Design review of the part shown in the three views and the two pictorial views. Dimensions are in mm from the part's minimum x, y and z. A direction names the side the tool comes from. Round coordinates to 2 decimals unless told otherwise and drop trailing zeros. Write each loop counter-clockwise with the first axis right and the second up, starting at its lowest first coordinate (ties: lowest second). Pieces come first, ordered by that corner, then holes. Notation, with made-up numbers: (25, 8) -> (83, 8) arc R24 cw to (83, 20) -> close; hole circle Ø4 at (8.5, 81.25). An arc over 180 degrees is marked (long way). Return JSON: item names as keys, results as strings. Group by question number.
1. Take a section at A-A, the plane z = 532.5. Write out the cut boundary in (x, y), then the cut area to 3 significant figures.
2. Take a section at D-D, the plane z = 832.5. Write out the cut boundary in (x, y), then the cut area to 3 significant figures.
3. Take a section at B-B, the plane y = 568.5. Write out the cut boundary in (x, z), then the cut area to 3 significant figures.
4. Clearance check with flat-ended pins moving along their axes: P1, Ø23, axis at x = 125.5, z = 437.5, coming from the +Y side; P2, Ø23, axis at y = 121.5, z = 427, coming from the -X side. State where each tip first meets the part, or that it passes through.
5. Mouldability with a two-part tool opening along Y and no side actions: class the marked faces 1, 2 and 3 as pulls with the +Y half, pulls with the -Y half, needs draft (parallel to the pull), parting line crosses it, or undercut.
6. Tool access review of the marked faces 4 and 5: name each direction out of +Z, -Z, +X, -X, +Y, -Y from which nothing blocks a thin tool from reaching the whole face with its end or side.
7. For line 1 along X through (y, z) = (1194, 764); line 2 along Y through (x, z) = (2033, 168); line 3 along X through (y, z) = (141, 113), list the stretches that pass through material, from the lowest coordinate up. Write a range as from..to.
8. Take a section at C-C, the plane x = 857. Write out the cut boundary in (y, z), then the cut area to 3 significant figures.
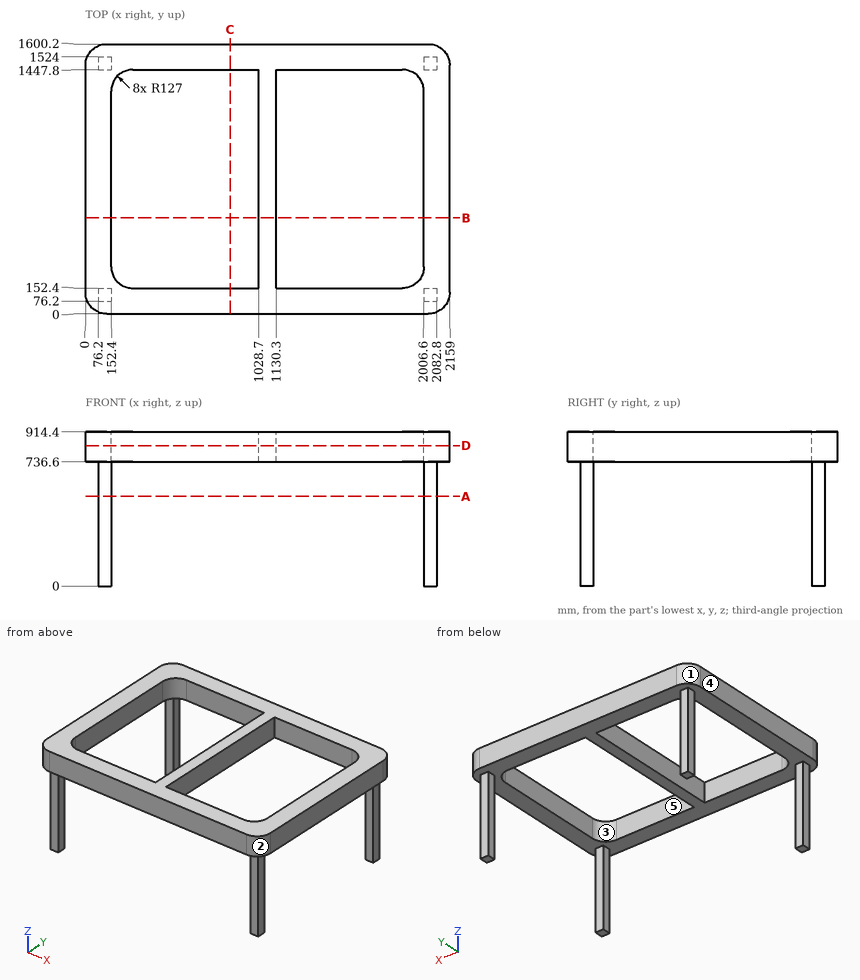
Output:
{
 "1": {"outline": "(76.2, 76.2) -> (152.4, 76.2) -> (152.4, 152.4) -> (76.2, 152.4) -> close; (76.2, 1447.8) -> (152.4, 1447.8) -> (152.4, 1524) -> (76.2, 1524) -> close; (2006.6, 76.2) -> (2082.8, 76.2) -> (2082.8, 152.4) -> (2006.6, 152.4) -> close; (2006.6, 1447.8) -> (2082.8, 1447.8) -> (2082.8, 1524) -> (2006.6, 1524) -> close", "area": "23,200 mm^2"},
 "2": {"outline": "(0, 127) arc R127 ccw to (127, 0) -> (2032, 0) arc R127 ccw to (2159, 127) -> (2159, 1473.2) arc R127 ccw to (2032, 1600.2) -> (127, 1600.2) arc R127 ccw to (0, 1473.2) -> close; hole (152.4, 279.4) arc R127 ccw to (279.4, 152.4) -> (1028.7, 152.4) -> (1028.7, 1447.8) -> (279.4, 1447.8) arc R127 ccw to (152.4, 1320.8) -> close; hole (1130.3, 152.4) -> (1879.6, 152.4) arc R127 ccw to (2006.6, 279.4) -> (2006.6, 1320.8) arc R127 ccw to (1879.6, 1447.8) -> (1130.3, 1447.8) -> close", "area": "1,180,000 mm^2"},
 "3": {"outline": "(0, 736.6) -> (152.4, 736.6) -> (152.4, 914.4) -> (0, 914.4) -> close; (1028.7, 736.6) -> (1130.3, 736.6) -> (1130.3, 914.4) -> (1028.7, 914.4) -> close; (2006.6, 736.6) -> (2159, 736.6) -> (2159, 914.4) -> (2006.6, 914.4) -> close", "area": "72,300 mm^2"},
 "4": {"P1": "stops at y = 1524", "P2": "stops at x = 76.2"},
 "5": {"face 1": "pulls with the +Y half", "face 2": "pulls with the -Y half", "face 3": "undercut"},
 "6": {"face 4": "+Z, -Z, -X, +Y, -Y", "face 5": "+Z, -Z"},
 "7": {"line 1": "x = 0..152.4, 1028.7..1130.3, 2006.6..2159", "line 2": "y = 76.2..152.4, 1447.8..1524", "line 3": "x = 76.2..152.4, 2006.6..2082.8"},
 "8": {"outline": "(0, 736.6) -> (152.4, 736.6) -> (152.4, 914.4) -> (0, 914.4) -> close; (1447.8, 736.6) -> (1600.2, 736.6) -> (1600.2, 914.4) -> (1447.8, 914.4) -> close", "area": "54,200 mm^2"}
}
